Source: CAD feature listing. Evaluate the final solid. Frame: model axes, mm. Face numbers are marked on the shaded views. Give positions to 0.01 mm unless a question says otherwise; leave off trailing zeros.
from build123d import *

# Parameters (mm, degrees)
PAD002_DEPTH    = 2
SKETCH016_R     = 2.5
POCKET001_DEPTH = 4
FILLET001_R     = 2


with BuildPart() as part:
    # Sketch013 → Pad002 (new body)
    with BuildSketch(Plane.XY):
        Polygon((17.320508, 10), (-17.320508, 10), (0, -20), align=None)
    extrude(amount=PAD002_DEPTH)

    # Sketch015 (on Face5 of Pad002) → AdditiveLoft004 section 0
    with BuildSketch(Plane.XY.offset(2)):
        Polygon((17.320508, 10), (-17.320508, 10), (0, -20), align=None)
    # Sketch014 (on Face5 of Pad002) → AdditiveLoft004 section 1
    with BuildSketch(Plane.XY.offset(12)):
        Polygon((0, -7), (6.062178, 3.5), (-6.062178, 3.5), align=None)
    loft()

    # Sketch016 (on Face4 of AdditiveLoft004) → Pocket001 (cut)
    with BuildSketch(Plane(origin=(0, 0, 0), x_dir=(1, 0, 0), z_dir=(0, 0, -1))):
        Circle(SKETCH016_R)
    extrude(amount=-POCKET001_DEPTH, mode=Mode.SUBTRACT)

    # Fillet001
    fillet001_edges = [part.edges().sort_by_distance(p)[0] for p in [
        (11.691343, 6.75, 7),
        (0, 3.5, 12),
        (-3.031089, -1.75, 12),
        (-11.691343, 6.75, 7),
        (3.031089, -1.75, 12),
        (0, -13.5, 7),
    ]]
    fillet(fillet001_edges, radius=FILLET001_R)


solid = part.part
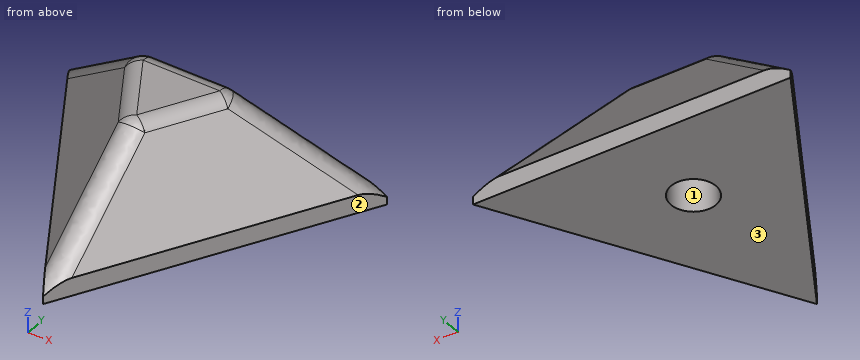
1) Ray query, L1, parallel to Y at x = 0, z = 1.2; L2, parallel to X at y = 0, z = 1.8; L3, parallel to Z at x = 2, y = 1. Return the intervals inside material, ascending.
Checks:
L1: y = -19.55 to -2.5, 2.5 to 10
L2: x = -11.55 to -2.5, 2.5 to 11.55
L3: z = 4 to 12
2) First-contact query: pin 1 Ø3 at (y, z) = (0, 2.5) entering from +X; pin 2 Ø5 at (y, z) = (-16, 4) entering from -X; pin 3 Ø5 at (y, z) = (3.5, 6) entering from +X; pin 4 Ø6 at (x, y) = (-5.5, -4) entering from -Z. Flat tips, straight axial feed; report the tip coordinate or a pass-through.
Checks:
pin 1: stops at x = 12.36
pin 2: stops at x = -3.18
pin 3: stops at x = 12.93
pin 4: stops at z = 0
3) Pull-direction query (X, two-part tool) for the marked faces 1, 2 and 3; classes: +X half, -X half, draft (parallel to the pull), parting line (faces both ways), or undercut.
Checks:
face 1: undercut
face 2: +X half
face 3: draft
